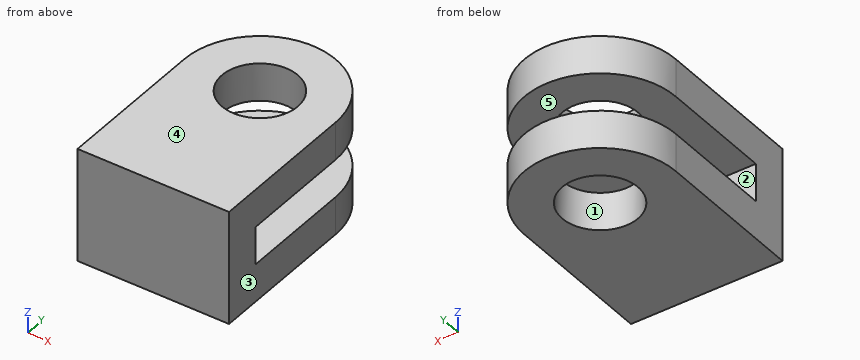
from build123d import *

# Parameters (mm, degrees)
SKETCH1_W           = 40
SKETCH1_H           = 10
BOSS_EXTRUDE1_DEPTH = 15
SKETCH1_3_R         = 10
BOSS_EXTRUDE2_DEPTH = 10


with BuildPart() as part:
    # Sketch1 → Boss-Extrude1 (new body)
    with BuildSketch(Plane.XY):
        with Locations((20, 5)):
            Rectangle(SKETCH1_W, SKETCH1_H)
    boss_extrude1 = extrude(amount=BOSS_EXTRUDE1_DEPTH)

    # Sketch1<3> → Boss-Extrude2 (add)
    with BuildSketch(Plane.XY):
        with BuildLine():
            Line((0, 40), (0, 10))
            Line((0, 10), (40, 10))
            Line((40, 10), (40, 40))
            ThreePointArc((40, 40), (20, 60), (0, 40))
        make_face()
        with Locations((20, 40)):
            Circle(SKETCH1_3_R, mode=Mode.SUBTRACT)
    boss_extrude2 = extrude(amount=BOSS_EXTRUDE2_DEPTH)

    # Mirror1: Boss-Extrude1, Boss-Extrude2 across plane
    add(boss_extrude1.mirror(Plane.XY.offset(15)))
    add(boss_extrude2.mirror(Plane.XY.offset(15)))


solid = part.part
Can you work these out from the model? Positions are in its coordinate system, mm. Face numbers are marked on the shaded views. A direction names the side the tool comes from. Give positions to 0.01 mm unless a question says otherwise; leave off trailing zeros. Loops run counter-clockwise (first coordinate to the right, second up) from the corner with the lowest first, then second, coordinate; pieces in that order, holes last. Notation, with made-up numbers: (14, -24) -> (45, -24) arc R22 cw to (45, 5) -> close; hole circle Ø4 at (60.5, 9). An arc over 180 degrees is marked (long way). Write item = value, one per line.
1) Suppose I cut it at D-D on z = 18. Write out the boundary of the cut face in (x, y).
Check result:
outline = (0, 0) -> (40, 0) -> (40, 10) -> (0, 10) -> close
2) Suppose I cut it at A-A on x = 20. Write out the boundary of the cut face in (y, z).
Check result:
outline = (0, 0) -> (30, 0) -> (30, 10) -> (10, 10) -> (10, 20) -> (30, 20) -> (30, 30) -> (0, 30) -> close; (50, 0) -> (60, 0) -> (60, 10) -> (50, 10) -> close; (50, 20) -> (60, 20) -> (60, 30) -> (50, 30) -> close
3) Will these pins go through, and if not, where does the flat tip stop? pin 1 (5 mm diameter, centred on x = 28, z = 5.5, fed in from +Y); pin 2 (5 mm diameter, centred on y = 54, z = 13, fed in from +X); pin 3 (11 mm diameter, centred on x = 16, z = 14, fed in from +Y); pin 4 (6 mm diameter, centred on y = 54, z = 19, fed in from +X).
Check result:
pin_1 = 59.23
pin_2 = through
pin_3 = 60
pin_4 = 36.59
4) Suppose I cut it at B-B on y = 22. Write out the boundary of the cut face in (x, z).
Check result:
outline = (0, 0) -> (40, 0) -> (40, 10) -> (0, 10) -> close; (0, 20) -> (40, 20) -> (40, 30) -> (0, 30) -> close
5) I need wall thicknesses on L1, parallel to Z at x = 15.5, y = 17.5; L2, parallel to Y at x = 20, z = 7.25; L3, parallel to Y at x = 15, z = 18. Which ranges of each line are inside material? Lowest first, please. Write a range as from..to.
Check result:
L1 = 0..10, 20..30
L2 = 0..30, 50..60
L3 = 0..10
6) Thinking about a two-plate mould opening in Z: for the marked faces 3, 4 and 5, which applies, released by +Z, released by -Z, zero draft, split by the parting line, or undercut?
Check result:
face_3 = zero draft
face_4 = released by +Z
face_5 = undercut
7) For the marked faces 1 and 2, which set-ups out of +Z, -Z, +X, -X, +Y, -Y let a thin tool reach every point of the face, with its end or its side?
Check result:
face_1 = +Z, -Z
face_2 = +X, -X, +Y
8) Suppose I cut it at C-C on z = 27.75. Write out the boundary of the cut face in (x, y).
Check result:
outline = (0, 0) -> (40, 0) -> (40, 40) arc R20 ccw to (0, 40) -> close; hole circle Ø20 at (20, 40)
